Source: three-view drawing plus pictorial views. Frame: mm from the lowest corner of the part. A direction names the side the tool comes from. Give positions to 0.01 mm unless a question says otherwise; leave off trailing zeros. Order: outer loops, then holes, each group sorted by start corner. A loop starts at its lowest first (then second) coordinate and runs counter-clockwise, first axis right, second up. Notation, with made-up numbers: M 67,-16 L 80,-16 A28 cw 80,16 Z; hole C 44.25,33.25 d11. An arc over 180 degrees is marked long. Use CSV: the item, a comma, the result in double quotes. Start each with the question number.
Item 1: First-contact query: pin 1 (2 mm diameter, centred on x = 3, y = 15, fed in from -Z). Flat tip, straight axial feed; report the tip coordinate or a pass-through.
Item 2: Ray query, probe 1 along X at (y, z) = (15.5, 67). Return the intervals inside material, ascending. Write a range as from..to.
Item 3: Access query for the marked faces 1 and 2. Directions: +Z, -Z, +X, -X, +Y, -Y. A direction counts if a zero-diameter tool reaches every point of the face in a straight line with its end or side. Return the directions, or none.
Item 4: Section query A-A on y = 3.75. Return loops of the section in (x, z).
Item 5: Section query C-C on z = 59.5. Return loops of the section in (x, y), and give its area (3 significant figures).
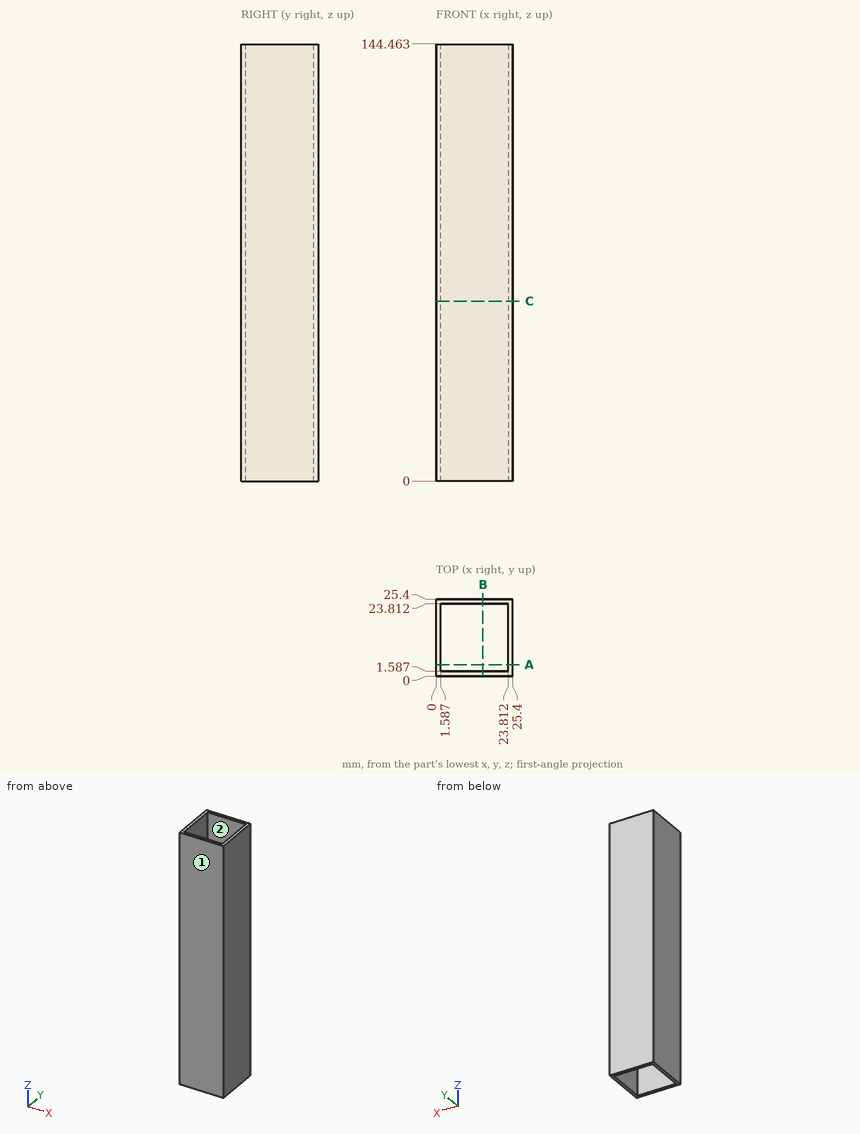
Verdict:
1,pin 1,"through"
2,probe 1,"0..1.59, 23.81..25.4"
3,face 1,"+Z, -Z, +X, -X, -Y"
3,face 2,"+Z, -Z"
4,outline,"M 0,0 L 1.59,0 L 1.59,144.46 L 0,144.46 Z; M 23.81,0 L 25.4,0 L 25.4,144.46 L 23.81,144.46 Z"
5,outline,"M 0,0 L 25.4,0 L 25.4,25.4 L 0,25.4 Z; hole M 1.59,1.59 L 23.81,1.59 L 23.81,23.81 L 1.59,23.81 Z"
5,area,"151 mm2"
